Verification items for this drawing (mm, ordinates from the low corner). Round coordinates to 2 decimals unless told otherwise and drop trailing zeros. Order: outer loops, then holes, each group sorted by start corner. A loop starts at its lowest first (then second) coordinate and runs counter-clockwise, first axis right, second up. Notation, with made-up numbers: (22, 59.25) -> (62, 59.25) arc R23 cw to (62, 67.25) -> close; hole circle Ø4 at (69, 16.25). An arc over 180 degrees is marked (long way). Return JSON: item names as keys, results as strings. Group by question number.
Item 1: Sectioned sample at A-A on x = 12. Record the cut outline in (y, z).
Item 2: Draft check along Y on the marked faces 1, 2 and 3. Enter one of: pulls with the +Y half, pulls with the -Y half, needs draft (parallel to the pull), parting line crosses it, or undercut.
Item 3: Depth check by flat-ended pin: pin 1 Ø4 at (y, z) = (6, 1.5) entering from +X; pin 2 Ø12 at (x, y) = (12, 11) entering from +Z; pin 3 Ø1 at (y, z) = (10, 3) entering from +X. Enter the tip coordinate at first touch or a pass-through.
Item 4: Scan lines: probe 1 along Y at (x, z) = (12, 3.75); probe 2 along X at (y, z) = (7.25, 4.75); probe 3 along Z at (x, y) = (5.5, 20.5). Record each from-to range of solid material in increasing order. Write a range as from..to.
Item 5: Sectioned sample at C-C on z = 3.25. Record the cut outline in (x, y).
Item 6: Sectioned sample at D-D on x = 22.5. Record the cut outline in (y, z), plus the area to 3 significant figures.
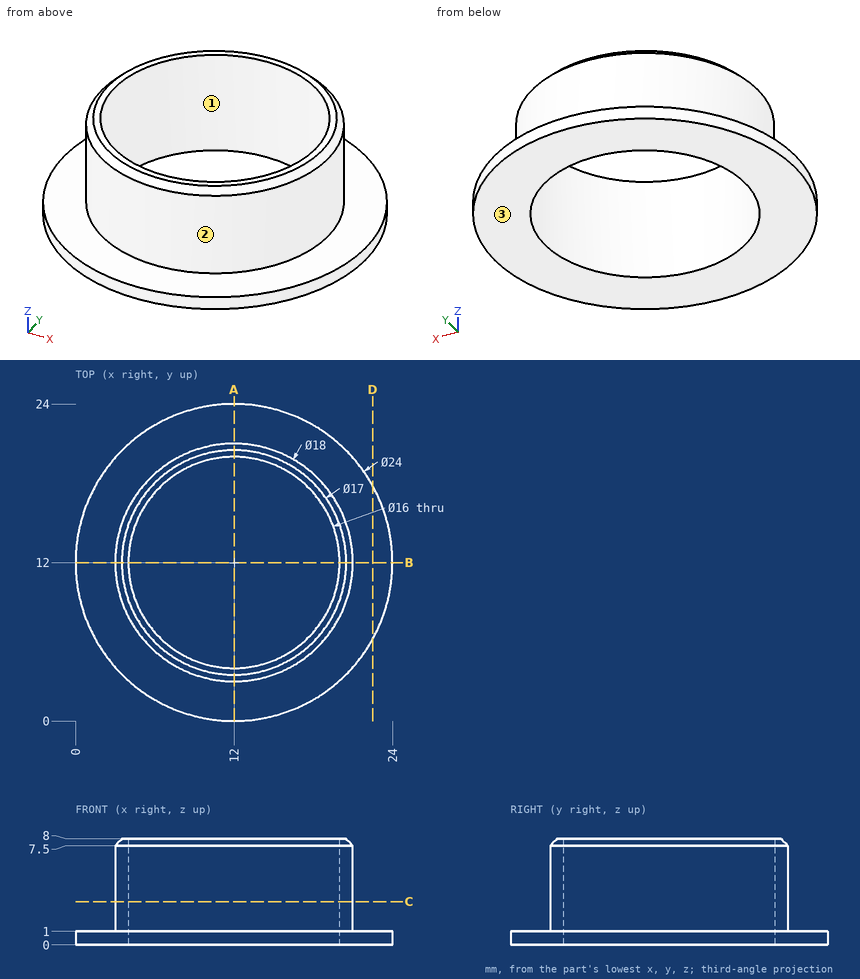
Recorded:
{
 "1": {"outline": "(0, 0) -> (4, 0) -> (4, 8) -> (3.5, 8) -> (3, 7.5) -> (3, 1) -> (0, 1) -> close; (20, 0) -> (24, 0) -> (24, 1) -> (21, 1) -> (21, 7.5) -> (20.5, 8) -> (20, 8) -> close"},
 "2": {"face 1": "undercut", "face 2": "parting line crosses it", "face 3": "needs draft"},
 "3": {"pin 1": "x = 23.29", "pin 2": "through", "pin 3": "x = 20.87"},
 "4": {"probe 1": "3..4, 20..21", "probe 2": "4.36..5.56, 18.44..19.64", "probe 3": "0..1"},
 "5": {"outline": "circle Ø18 at (12, 12); hole circle Ø16 at (12, 12)"},
 "6": {"outline": "(6.19, 0) -> (17.81, 0) -> (17.81, 1) -> (6.19, 1) -> close", "area": "11.6 mm²"}
}
